from build123d import *

# Parameters (mm, degrees)
F0_R           = 62.5
F1_DEPTH       = 3.95
F2_R           = 45
F3_DEPTH       = 4.05
F6_D           = 5
F6_DEPTH       = 24.25
F6_CBORE_D     = 11.25
F6_CBORE_DEPTH = 6
F6_TIP         = 1.5021515476


with BuildPart() as f1:
    # F0 (on Front) → F1 (new body)
    with BuildSketch(Plane.XZ):
        Circle(F0_R)
    extrude(amount=-F1_DEPTH)

    # F2 (on face) → F3 (join)
    with BuildSketch(Plane(origin=(0, 3.95, 0), x_dir=(-1, 0, 0), z_dir=(0, 1, 0))):
        Circle(F2_R)
    extrude(amount=F3_DEPTH)

    # F4 (on Top) → F5 (revolve, cut)
    with BuildSketch(Plane.XY):
        Polygon((0, 8), (0, 0), (25, 0), (18, 7), (18, 8), align=None)
    revolve(axis=Axis((0, 4, 0), (0, 1, 0)), mode=Mode.SUBTRACT)

    # F6
    with Locations(Plane.XZ):
        with Locations((37.5, 0), (0, -37.5), (-37.5, 0), (0, 37.5)):
            CounterBoreHole(F6_D / 2, F6_CBORE_D / 2, F6_CBORE_DEPTH, depth=F6_DEPTH)
            with Locations((0, 0, -(F6_DEPTH + F6_TIP / 2))):  # 118° drill point
                Cone(0, F6_D / 2, F6_TIP, mode=Mode.SUBTRACT)


solid = f1.part
Verification items for the finished model (mm, model axes). A direction names the side the tool comes from. Round coordinates to 2 decimals unless told otherwise and drop trailing zeros. Order: outer loops, then holes, each group sorted by start corner. A loop starts at its lowest first (then second) coordinate and runs counter-clockwise, first axis right, second up.
1. Section check D-D on x = -37.5. Record the cut outline in (y, z) (3 decimals).
Final values:
outline: (0, -50) - (3.95, -50) - (3.95, -24.875) - (8, -24.875) - (8, -2.5) - (6, -2.5) - (6, -5.625) - (0, -5.625) - close; (0, 5.625) - (6, 5.625) - (6, 2.5) - (8, 2.5) - (8, 24.875) - (3.95, 24.875) - (3.95, 50) - (0, 50) - close
2. Access from +Z, -Z, +X, -X, +Y, -Y to the whole of each face (thin tool, end or side, straight path). Record for faces 1 (the cylindrical face through (-62.44, 1.95, 2.75)), 2 (the flat face through (40, 6, -1)), 3 (the flat face through (-43, 3.95, 15)).
Final values:
face 1: +Y, -Y
face 2: -Y
face 3: +Y
3. Section check A-A on x = 0. State how many separate pieces and enclosed holes the cut face has, then the cut area to 3 significant figures.
Final values:
separate pieces: 4
enclosed holes: 0
area: 366 mm2
4. Section check B-B on y = 2.25. Record the cut outline in (x, z) (3 decimals).
Final values:
outline: circle Ø125 at (0, 0); hole circle Ø11.25 at (-37.5, 0); hole circle Ø45.5 at (0, 0); hole circle Ø11.25 at (0, -37.5); hole circle Ø11.25 at (0, 37.5); hole circle Ø11.25 at (37.5, 0)
5. Go/stop test with flat-tipped pins: P1, Ø7, axis at x = -37.5, z = 0, coming from the -Y side; P2, Ø1.5, axis at y = 2.5, z = -44.5, coming from the -X side; P3, Ø1.5, axis at y = 1.5, z = 9.5, coming from the +X side. Record where each tip stops, or that it passes through.
Final values:
P1: stops at y = 6
P2: stops at x = -44.63
P3: stops at x = 61.88
6. Thickness scan on L1, parallel to Z at x = 0, y = 7.7; L2, parallel to Y at x = -43, z = -34; L3, parallel to Z at x = 0, y = 1.8 (3 decimals). Record the ranges inside material, lowest first.
Final values:
L1: z = -45 to -40, -35 to -18, 18 to 35, 40 to 45
L2: y = 0 to 3.95
L3: z = -62.5 to -43.125, -31.875 to -23.2, 23.2 to 31.875, 43.125 to 62.5
7. Section check C-C on z = 37.5. Record the cut outline in (x, y) (3 decimals), then the cut area to 3 significant figures.
Final values:
outline: (-50, 0) - (-5.625, 0) - (-5.625, 6) - (-2.5, 6) - (-2.5, 8) - (-24.875, 8) - (-24.875, 3.95) - (-50, 3.95) - close; (2.5, 6) - (5.625, 6) - (5.625, 0) - (50, 0) - (50, 3.95) - (24.875, 3.95) - (24.875, 8) - (2.5, 8) - close
area: 519 mm2
